Verification items for the finished model (mm, model axes). A direction names the side the tool comes from. Round coordinates to 2 decimals unless told otherwise and drop trailing zeros. Write each loop counter-clockwise with the first axis right and the second up, starting at its lowest first coordinate (ties: lowest second). Pieces come first, ordered by that corner, then holes.
from build123d import *

# Parameters (mm, degrees)
SKETCH_R     = 13.5
SKETCH_R_2   = 1.75
PAD_DEPTH    = 4
SKETCH004_W  = 28.8
SKETCH004_H  = 2
PAD001_DEPTH = 6
SKETCH005_R  = 4
POCKET_DEPTH = 3
SKETCH006_W  = 5
SKETCH006_H  = 10
PAD002_DEPTH = 10
FILLET_R     = 9.9


with BuildPart() as part:
    # Sketch → Pad (new body)
    with BuildSketch(Plane.XY):
        Circle(SKETCH_R)
        with Locations((-5.656854, -5.656854)):
            Circle(SKETCH_R_2, mode=Mode.SUBTRACT)
        with Locations((5.656854, 5.656854)):
            Circle(SKETCH_R_2, mode=Mode.SUBTRACT)
        with Locations((-5.656854, 5.656854)):
            Circle(SKETCH_R_2, mode=Mode.SUBTRACT)
        with Locations((5.656854, -5.656854)):
            Circle(SKETCH_R_2, mode=Mode.SUBTRACT)
    extrude(amount=PAD_DEPTH)

    # Sketch004 → Pad001 (join)
    with BuildSketch(Plane(origin=(0, 0, 0), x_dir=(1, 0, 0), z_dir=(0, 0, -1))):
        Rectangle(SKETCH004_W, SKETCH004_H)
    extrude(amount=-PAD001_DEPTH)

    # Sketch005 (on Face1 of Pad001) → Pocket (cut)
    with BuildSketch(Plane(origin=(0, 0, 0), x_dir=(1, 0, 0), z_dir=(0, 0, -1))):
        Circle(SKETCH005_R)
    extrude(amount=-POCKET_DEPTH, mode=Mode.SUBTRACT)

    # Sketch006 (on Face18 of Pocket) → Pad002 (join)
    with BuildSketch(Plane.XY.offset(4)):
        with Locations((0, -7.6)):
            Rectangle(SKETCH006_W, SKETCH006_H)
        with Locations((0, 7.6)):
            Rectangle(SKETCH006_W, SKETCH006_H)
    extrude(amount=PAD002_DEPTH)

    # Fillet
    fillet_edges = [part.edges().sort_by_distance(p)[0] for p in [
        (0, 12.6, 14),
        (0, -12.6, 14),
    ]]
    fillet(fillet_edges, radius=FILLET_R)


solid = part.part
Q1. Release check for a two-part mould opening along Y. For faces 1 (the cylindrical face through (0, -9.8, 11)), 2 (the flat face through (0, 2.6, 9)), 3 (the flat face through (14.4, 0, 3)) record: released by +Y, released by -Y, zero draft, split by the parting line, or undercut.
Recorded:
face 1: released by -Y
face 2: undercut
face 3: zero draft
Q2. Sectioned sample at B-B (x = 0). Enter the section's corners in (y, z).
Recorded:
outline: (-13.5, 0) - (-4, 0) - (-4, 3) - (4, 3) - (4, 0) - (13.5, 0) - (13.5, 4) - (12.6, 4) - (12.6, 4.1) arc R9.9 ccw to (2.7, 14) - (2.6, 14) - (2.6, 4) - (1, 4) - (1, 6) - (-1, 6) - (-1, 4) - (-2.6, 4) - (-2.6, 14) - (-2.7, 14) arc R9.9 ccw to (-12.6, 4.1) - (-12.6, 4) - (-13.5, 4) - close
Q3. Sectioned sample at D-D (y = -6). Enter the section's corners in (x, z).
Recorded:
outline: (-12.09, 0) - (-7.37, 0) - (-7.37, 4) - (-12.09, 4) - close; (-3.94, 0) - (3.94, 0) - (3.94, 4) - (2.5, 4) - (2.5, 13.43) - (-2.5, 13.43) - (-2.5, 4) - (-3.94, 4) - close; (7.37, 0) - (12.09, 0) - (12.09, 4) - (7.37, 4) - close
Q4. Depth check by flat-ended pin: P1, Ø5, axis at x = -7, y = -1, coming from the +Z side; P2, Ø4, axis at x = 4, y = 6.5, coming from the +Z side; P3, Ø3, axis at y = -6.5, z = 1.5, coming from the +X side. Enter the tip coordinate at first touch or a pass-through.
Recorded:
P1: stops at z = 6
P2: stops at z = 13.69
P3: stops at x = 12.54
Q5. Material ranges on line 1 along Y through (x, z) = (5.25, 2.5); line 2 along Z through (x, y) = (4.75, 3.5); line 3 along Z through (x, y) = (2.5, 0.25), recorded low to high.
Recorded:
line 1: y = -12.44 to -7.36, -3.95 to 3.95, 7.36 to 12.44
line 2: z = 0 to 4
line 3: z = 3 to 6
Q6. Tool access check on faces 4 (the cylindrical face through (-0.867, 3.905, 1.479)), 5 (the flat face through (2.5, -7, 8)), 6 (the flat face through (0, -2.6, 9)), 7 (the flat face through (-2.5, 6, 8)). Record the directions out of +Z, -Z, +X, -X, +Y, -Y that give a thin tool (end or side, any length) a straight path to the whole face; none if there is none.
Recorded:
face 4: -Z
face 5: +Z, +X, -Y
face 6: +Z, +X, -X
face 7: +Z, -X, +Y
Q7. Sectioned sample at C-C (z = 11.75). Enter the section's corners in (x, y), plus the area to 3 significant figures.
Recorded:
outline: (-2.5, -8.98) - (2.5, -8.98) - (2.5, -2.6) - (-2.5, -2.6) - close; (-2.5, 2.6) - (2.5, 2.6) - (2.5, 8.98) - (-2.5, 8.98) - close
area: 63.8 mm2
Q8. Sectioned sample at A-A (z = 5.5). Enter the section's corners in (x, y).
Recorded:
outline: (-14.4, -1) - (14.4, -1) - (14.4, 1) - (-14.4, 1) - close; (-2.5, -12.5) - (2.5, -12.5) - (2.5, -2.6) - (-2.5, -2.6) - close; (-2.5, 2.6) - (2.5, 2.6) - (2.5, 12.5) - (-2.5, 12.5) - close
